```python
from build123d import *

# Parameters (mm, degrees)
TUBE_SQUARE_40_X_40_X_3_2_5_DEPTH = 1960
CUT_EXTRUDE1_DEPTH                = 1961.510137694
SKETCH15_R                        = 2
CUT_EXTRUDE3_DEPTH                = 1961.204071009


with BuildPart() as part:
    # Sketch12 → Tube (square) 40 X 40 X 3.2(5) (new body)
    with BuildSketch(Plane(origin=(0, 0, 0), x_dir=(0, 0, -1), z_dir=(1, 0, 0))):
        with BuildLine():
            Line((-13.6, -20), (13.6, -20))
            ThreePointArc((13.6, -20), (18.1254834, -18.1254834), (20, -13.6))
            Line((20, -13.6), (20, 13.6))
            ThreePointArc((20, 13.6), (18.1254834, 18.1254834), (13.6, 20))
            Line((13.6, 20), (-13.6, 20))
            ThreePointArc((-13.6, 20), (-18.1254834, 18.1254834), (-20, 13.6))
            Line((-20, 13.6), (-20, -13.6))
            ThreePointArc((-20, -13.6), (-18.1254834, -18.1254834), (-13.6, -20))
        make_face()
        with BuildLine():
            Line((-13.6, -16.8), (13.6, -16.8))
            ThreePointArc((13.6, -16.8), (15.8627417, -15.8627417), (16.8, -13.6))
            Line((16.8, -13.6), (16.8, 13.6))
            ThreePointArc((16.8, 13.6), (15.8627417, 15.8627417), (13.6, 16.8))
            Line((13.6, 16.8), (-13.6, 16.8))
            ThreePointArc((-13.6, 16.8), (-15.8627417, 15.8627417), (-16.8, 13.6))
            Line((-16.8, 13.6), (-16.8, -13.6))
            ThreePointArc((-16.8, -13.6), (-15.8627417, -15.8627417), (-13.6, -16.8))
        make_face(mode=Mode.SUBTRACT)
    extrude(amount=TUBE_SQUARE_40_X_40_X_3_2_5_DEPTH)

    # Sketch13 → Cut-Extrude1 (cut, through all)
    with BuildSketch(Plane(origin=(0, 20, 0), x_dir=(1, 0, 0), z_dir=(0, 1, 0))):
        Polygon((1960, 20), (1960, -20), (1920, 20), align=None)
        Polygon((0, 20), (0, -20), (40, 20), align=None)
    extrude(amount=-CUT_EXTRUDE1_DEPTH, mode=Mode.SUBTRACT)

    # Sketch15 → Cut-Extrude3 (cut, through all)
    with BuildSketch(Plane(origin=(0, 0, 0), x_dir=(1, 0, 0), z_dir=(0, 1, 0))):
        with Locations(Location((980, 0, 0), (0, 0, 270))):
            Circle(SKETCH15_R)
        with Locations((20, 0)):
            Circle(SKETCH15_R)
        with Locations((1940, 0)):
            Circle(SKETCH15_R)
        with Locations(Location((500, 0, 0), (0, 0, 270))):
            Circle(SKETCH15_R)
        with Locations(Location((1460, 0, 0), (0, 0, 270))):
            Circle(SKETCH15_R)
    extrude(amount=-CUT_EXTRUDE3_DEPTH, mode=Mode.SUBTRACT)


solid = part.part
```
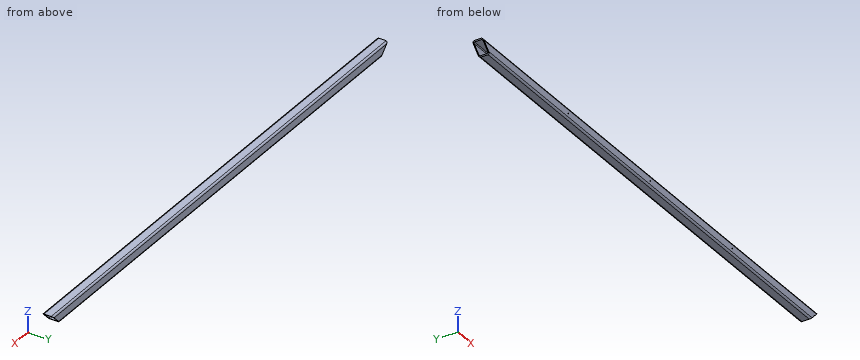
Geometry check sheet. Reference: the model listing, model coordinates, mm. Round coordinates to 2 decimals unless told otherwise and drop trailing zeros. Write each loop counter-clockwise with the first axis right and the second up, starting at its lowest first coordinate (ties: lowest second). Pieces come first, ordered by that corner, then holes. Notation, with made-up numbers: (86, 4) - (127, 4) arc R31 cw to (127, 29) - close; hole circle Ø11 at (23.5, 60). An arc over 180 degrees is marked (long way). Write each question's results on one line, items separated by ' | '.
(1) Sectioned sample at A-A, the plane y = 2. Enter the section's corners in (x, z).
Computed:
outline: (0, 20) - (3.2, 16.8) - (1956.8, 16.8) - (1960, 20) - close; (36.8, -16.8) - (40, -20) - (1920, -20) - (1923.2, -16.8) - close
(2) Sectioned sample at B-B, the plane x = 653.5. Enter the section's corners in (y, z).
Computed:
outline: (-20, -13.6) arc R6.4 ccw to (-13.6, -20) - (13.6, -20) arc R6.4 ccw to (20, -13.6) - (20, 13.6) arc R6.4 ccw to (13.6, 20) - (-13.6, 20) arc R6.4 ccw to (-20, 13.6) - close; hole (-16.8, -13.6) arc R3.2 ccw to (-13.6, -16.8) - (13.6, -16.8) arc R3.2 ccw to (16.8, -13.6) - (16.8, 13.6) arc R3.2 ccw to (13.6, 16.8) - (-13.6, 16.8) arc R3.2 ccw to (-16.8, 13.6) - close
(3) Depth check by flat-ended pin: pin 1 Ø6 at (x, y) = (1425, 14) entering from +Z; pin 2 Ø10 at (y, z) = (12.5, 9.5) entering from -X; pin 3 Ø3.5 at (x, z) = (500, 0) entering from -Y; pin 4 Ø12 at (y, z) = (14.5, 0.5) entering from +X. Enter the tip coordinate at first touch or a pass-through.
Computed:
pin 1: stops at z = 20 | pin 2: stops at x = 7.95 | pin 3: stops at y = 16.8 | pin 4: stops at x = 1946.04
(4) Thickness scan on probe 1 along X at (y, z) = (-17.55, 0); probe 2 along Y at (x, z) = (1037, 10). Record the ranges inside material, lowest first. Write a range as from..to.
Computed:
probe 1: x = 22..498, 502..978, 982..1458, 1462..1938 | probe 2: y = -20..-16.8, 16.8..20
